Verification items for this drawing (mm, ordinates from the low corner). Coordinates: 2 decimals unless noted, no trailing zeros. Write each loop counter-clockwise with the first axis right and the second up, starting at its lowest first coordinate (ties: lowest second). Pieces come first, ordered by that corner, then holes.
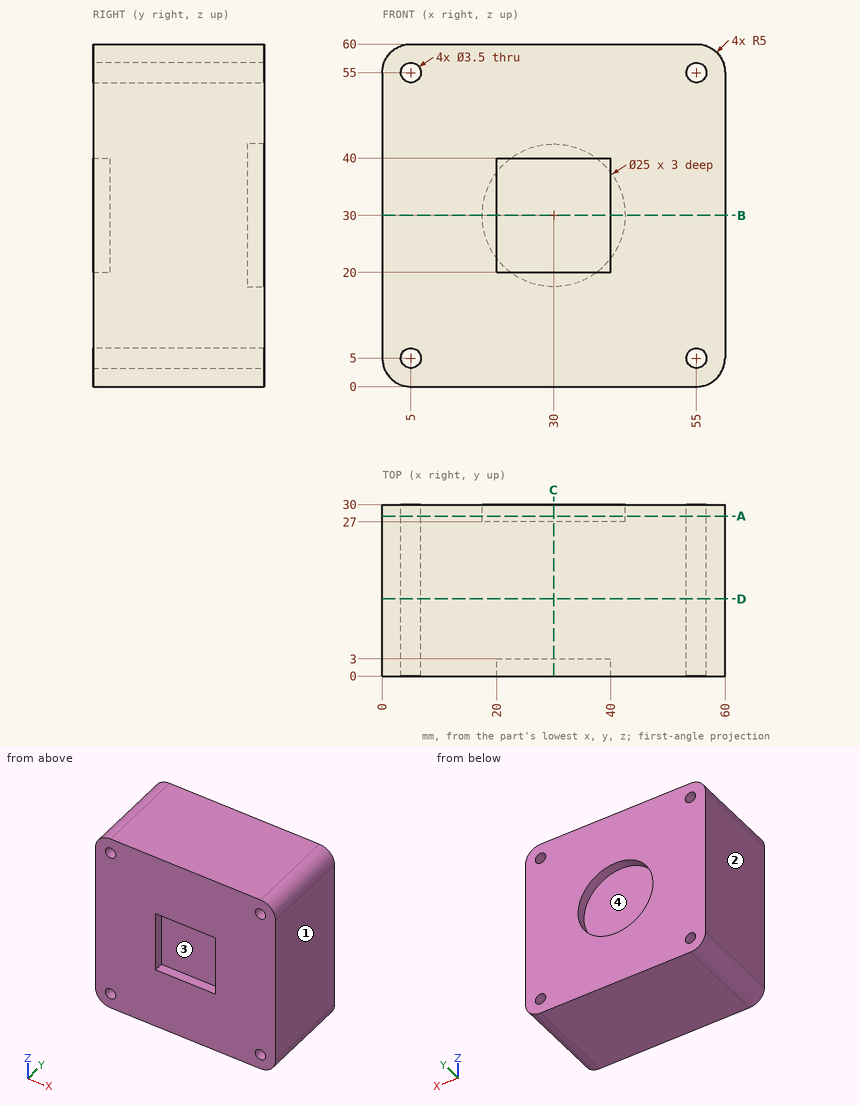
1. Thickness scan on line 1 along X through (y, z) = (18.25, 55); line 2 along X through (y, z) = (29.25, 30); line 3 along Z through (x, y) = (4, 10.75). Record the ranges inside material, lowest first.
Computed values:
line 1: x = 0 to 3.25, 6.75 to 53.25, 56.75 to 60
line 2: x = 0 to 17.5, 42.5 to 60
line 3: z = 0.1 to 3.56, 6.44 to 53.56, 56.44 to 59.9
2. Sectioned sample at B-B, the plane z = 30. Record the boundary of the cut face in (x, y), and give its area (4 significant figures).
Computed values:
outline: (0, 0) - (20, 0) - (20, 3) - (40, 3) - (40, 0) - (60, 0) - (60, 30) - (42.5, 30) - (42.5, 27) - (17.5, 27) - (17.5, 30) - (0, 30) - close
area: 1,665 mm2
3. Gauge pin test, flat ends, axial feed: pin 1 Ø22.5 at (x, z) = (30, 30) entering from -Y; pin 2 Ø2 at (x, z) = (38.5, 32) entering from +Y; pin 3 Ø6 at (x, z) = (26, 31.5) entering from -Y. Record the tip position at first contact, or that the pin passes through.
Computed values:
pin 1: stops at y = 0
pin 2: stops at y = 27
pin 3: stops at y = 3
4. Sectioned sample at C-C, the plane x = 30. Record the boundary of the cut face in (y, z), and give its area (4 significant figures).
Computed values:
outline: (0, 0) - (30, 0) - (30, 17.5) - (27, 17.5) - (27, 42.5) - (30, 42.5) - (30, 60) - (0, 60) - (0, 40) - (3, 40) - (3, 20) - (0, 20) - close
area: 1,665 mm2
5. Draft check along X on the marked faces 1, 2, 3 and 4. Enter one of: released by +X, released by -X, zero draft, split by the parting line, or undercut.
Computed values:
face 1: released by +X
face 2: released by -X
face 3: undercut
face 4: undercut
6. Sectioned sample at A-A, the plane y = 28. Record the boundary of the cut face in (x, z), and give its area (3 significant figures).
Computed values:
outline: (0, 5) arc R5 ccw to (5, 0) - (55, 0) arc R5 ccw to (60, 5) - (60, 55) arc R5 ccw to (55, 60) - (5, 60) arc R5 ccw to (0, 55) - close; hole circle Ø3.5 at (5, 5); hole circle Ø3.5 at (5, 55); hole circle Ø25 at (30, 30); hole circle Ø3.5 at (55, 5); hole circle Ø3.5 at (55, 55)
area: 3,050 mm2
7. Sectioned sample at D-D, the plane y = 13.5. Record the boundary of the cut face in (x, z).
Computed values:
outline: (0, 5) arc R5 ccw to (5, 0) - (55, 0) arc R5 ccw to (60, 5) - (60, 55) arc R5 ccw to (55, 60) - (5, 60) arc R5 ccw to (0, 55) - close; hole circle Ø3.5 at (5, 5); hole circle Ø3.5 at (5, 55); hole circle Ø3.5 at (55, 5); hole circle Ø3.5 at (55, 55)
